```python
from build123d import *

# Parameters (mm, degrees)
ESBO_O1_R                = 50
RESSALTO_EXTRUS_O1_DEPTH = 1.6
ESBO_O2_R                = 1.6
CORTE_EXTRUS_O1_DEPTH    = 71.728777736


with BuildPart() as part:
    # Esboço1 → Ressalto-extrusão1 (new body)
    with BuildSketch(Plane(origin=(0, 0, 0), x_dir=(1, 0, 0), z_dir=(0, 1, 0))):
        with Locations(Location((0, 0, 0), (0, 0, 270))):
            Circle(ESBO_O1_R)
    extrude(amount=RESSALTO_EXTRUS_O1_DEPTH)

    # Esboço2 → Corte-extrusão1 (cut, through all)
    with BuildSketch(Plane.XZ):
        with Locations(Location((-30.0520382, -30.0520382, 0), (0, 0, 270))):
            Circle(ESBO_O2_R)
        with Locations(Location((-30.0520382, 30.0520382, 0), (0, 0, 270))):
            Circle(ESBO_O2_R)
        with Locations(Location((30.0520382, 30.0520382, 0), (0, 0, 270))):
            Circle(ESBO_O2_R)
        with Locations(Location((30.0520382, -30.0520382, 0), (0, 0, 270))):
            Circle(ESBO_O2_R)
    extrude(amount=-CORTE_EXTRUS_O1_DEPTH, mode=Mode.SUBTRACT)


solid = part.part
```
For this review, take the finished solid that the model builds, in its own axes (mm). Coordinates: 2 decimals unless noted, no trailing zeros. Write each loop counter-clockwise with the first axis right and the second up, starting at its lowest first coordinate (ties: lowest second). Pieces come first, ordered by that corner, then holes. Notation, with made-up numbers: (43.5, -32) -> (73.5, -32) arc R21 ccw to (73.5, 4) -> close; hole circle Ø7 at (77.5, 67.5). An arc over 180 degrees is marked (long way). Put each result on its own line as item: value.
Q1. Take a section at C-C, the plane y = 0.5. State the section outline as (x, z) points, then the cut area to 3 significant figures.
From the geometry:
outline: circle Ø100 at (0, 0); hole circle Ø3.2 at (-30.05, -30.05); hole circle Ø3.2 at (-30.05, 30.05); hole circle Ø3.2 at (30.05, -30.05); hole circle Ø3.2 at (30.05, 30.05)
area: 7,820 mm2
Q2. The part is to be moulded in two halves that separate along X. For faces 1 (the cylindrical face through (-28.466, 0.789, 30.26)), 2 (the cylindrical face through (28.49, 0.79, 30.4)), 3 (the flat face through (1, 0, -1)), 4 (the cylindrical face through (15.02, 0.79, 47.69)), say which applies: +X half, -X half, draft (parallel to the pull), parting line (faces both ways), or undercut.
From the geometry:
face 1: undercut
face 2: undercut
face 3: draft
face 4: parting line
Q3. Take a section at D-D, the plane x = 13. State the section outline as (y, z) points.
From the geometry:
outline: (0, -48.28) -> (1.6, -48.28) -> (1.6, 48.28) -> (0, 48.28) -> close
Q4. Take a section at A-A, the plane z = 30. State the section outline as (x, y) points, then the cut area to 3 significant figures.
From the geometry:
outline: (-40, 0) -> (-31.65, 0) -> (-31.65, 1.6) -> (-40, 1.6) -> close; (-28.45, 0) -> (28.45, 0) -> (28.45, 1.6) -> (-28.45, 1.6) -> close; (31.65, 0) -> (40, 0) -> (40, 1.6) -> (31.65, 1.6) -> close
area: 118 mm2
Q5. Take a section at B-B, the plane z = -14. State the section outline as (x, y) points.
From the geometry:
outline: (-48, 0) -> (48, 0) -> (48, 1.6) -> (-48, 1.6) -> close
Q6. Wall thickness on L1, parallel to X at y = 0.45, z = 24; L2, parallel to Z at x = 2, y = 1.4; L3, parallel to Z at x = 13, y = 0.4: over which ranges is each line inside the solid? List them lowest first.
From the geometry:
L1: x = -43.86 to 43.86
L2: z = -49.96 to 49.96
L3: z = -48.28 to 48.28
